from build123d import *

# Parameters (mm, degrees)
F0_R     = 41.275
F1_DEPTH = 88.9
F2_R     = 50.8
F2_R_2   = 41.275
F3_DEPTH = 12.7
F5_DEPTH = 76.2
F6_R     = 38.1
F7_DEPTH = 76.2


with BuildPart() as f1:
    # F0 (on Right) → F1 (new body)
    with BuildSketch(Plane.YZ):
        Circle(F0_R)
    extrude(amount=F1_DEPTH)

    # F2 (on face) → F3 (join)
    with BuildSketch(Plane.YZ.offset(88.9)):
        Circle(F2_R)
        Circle(F2_R_2, mode=Mode.SUBTRACT)
    extrude(amount=-F3_DEPTH)

    # F4 (on face) → F5 (cut)
    with BuildSketch(Plane.YZ):
        with BuildLine():
            Line((6.35, -21.4923172526), (-6.35, -21.4923172526))
            Line((-6.35, -21.4923172526), (-6.35, -40.7836134373))
            ThreePointArc((-6.35, -40.7836134373), (0, -41.275), (6.35, -40.7836134373))
            Line((6.35, -40.7836134373), (6.35, -21.4923172526))
        make_face()
    extrude(amount=F5_DEPTH, mode=Mode.SUBTRACT)

    # F6 (on face) → F7 (cut)
    with BuildSketch(Plane.YZ):
        Circle(F6_R)
    extrude(amount=F7_DEPTH, mode=Mode.SUBTRACT)


solid = f1.part
Can you work these out from the model? Positions are in its coordinate system, mm. A direction names the side the tool comes from. Coordinates: 2 decimals unless noted, no trailing zeros. Write each loop counter-clockwise with the first axis right and the second up, starting at its lowest first coordinate (ties: lowest second). Pieces come first, ordered by that corner, then holes. Notation, with made-up numbers: (33, -26) -> (70, -26) arc R16 cw to (70, -17) -> close; hole circle Ø4 at (5.25, -36). An arc over 180 degrees is marked (long way). Write each question's results on one line, items separated by ' | '. Start each with the question number.
Q1. I'm going to push flat-ended pins straight in: pin 1 (3.5 mm diameter, centred on x = 56, z = -39.5, fed in from -Y); pin 2 (1.5 mm diameter, centred on x = 72.5, y = -36, fed in from +Z); pin 3 (1.5 mm diameter, centred on x = 40, y = -35.5, fed in from -Z). Where does each tip first touch, or does it pass through?
Q2. On a 3-axis mill with a long thin cutter (end or side, diameter ignored), from which of +Z, -Z, +X, -X, +Y, -Y can I reach the whole of each face in a straight line? I mean faces 1 (the face through (38, -6.35, -39)), 2 (the face through (82.639, -11.012, -49.592)), 3 (the face through (37.567, 1.586, 38.067)). Say none if no direction works.
Q3. Imagine slicing it at D-D (z = 24). Write out the boundary of the cut face in (x, y), then the cut area to 3 significant figures.
Q4. If I drill on probe 1 along Y at (x, z) = (46, 0) (3 decimals); probe 2 along Z at (x, y) = (51.5, 0) (3 decimals); probe 3 along X at (y, z) = (-13, 41.5), over which ranges is the centre line in solid material (lowest first)?
Q5. Imagine slicing it at A-A (z = 0). Write out the boundary of the cut face in (x, y) (3 decimals).
Q6. We'd pull the mould along Z, two halves only. Please class faces 4 (the face through (0, 33.4, 18.7)), 5 (the face through (76.2, -1, 1)), 6 (the face through (37.57, 1.73, 41.24)): +Z half, -Z half, draft (parallel to the pull), parting line (faces both ways), or undercut.
Q7. Imagine slicing it at B-B (y = 0). Write out the boundary of the cut face in (x, z) (3 decimals), then the cut area to 3 significant figures.
Q8. Imagine slicing it at C-C (x = 71). Write out the boundary of the cut face in (y, z) (3 decimals).
Taken from the geometry:
1) pin 1: stops at y = -16.69 | pin 2: stops at z = 21.47 | pin 3: stops at z = -22.27
2) face 1: -Z, -X | face 2: +X, -X | face 3: -X
3) outline: (0, -33.58) -> (76.2, -33.58) -> (76.2, -44.77) -> (88.9, -44.77) -> (88.9, 44.77) -> (76.2, 44.77) -> (76.2, 33.58) -> (0, 33.58) -> (0, 29.59) -> (76.2, 29.59) -> (76.2, -29.59) -> (0, -29.59) -> close | area: 1,750 mm^2
4) probe 1: y = -41.275 to -38.1, 38.1 to 41.275 | probe 2: z = 38.1 to 41.275 | probe 3: x = 76.2 to 88.9
5) outline: (0, -41.275) -> (76.2, -41.275) -> (76.2, -50.8) -> (88.9, -50.8) -> (88.9, 50.8) -> (76.2, 50.8) -> (76.2, 41.275) -> (0, 41.275) -> (0, 38.1) -> (76.2, 38.1) -> (76.2, -38.1) -> (0, -38.1) -> close
6) face 4: draft | face 5: undercut | face 6: parting line
7) outline: (0, 38.1) -> (76.2, 38.1) -> (76.2, -50.8) -> (88.9, -50.8) -> (88.9, 50.8) -> (76.2, 50.8) -> (76.2, 41.275) -> (0, 41.275) -> close | area: 1,530 mm^2
8) outline: (-6.35, -40.784) -> (-6.35, -37.567) arc R38.1 cw (long way) to (6.35, -37.567) -> (6.35, -40.784) arc R41.275 ccw (long way) to start
